For this review, take the finished solid that the model builds, in its own axes (mm). A direction names the side the tool comes from. Give positions to 0.01 mm unless a question says otherwise; leave off trailing zeros. Loops run counter-clockwise (first coordinate to the right, second up) from the corner with the lowest first, then second, coordinate; pieces in that order, holes last. Notation, with made-up numbers: (-36.75, 33.25) - (6.25, 33.25) arc R16 cw to (6.25, 53.25) - close; hole circle Ø11 at (81.5, 23). An arc over 180 degrees is marked (long way). Answer in a Markdown table with one row per item.
```python
from build123d import *

# Parameters (mm, degrees)
F0_W     = 20
F0_H     = 20
F1_DEPTH = 10
F2_R     = 2.5
F3_DEPTH = 2
F4_R     = 2.5
F5_DEPTH = 2
F6_R     = 2.5
F7_DEPTH = 2
F8_R     = 1.5


# Not quite as in the source:
# - a pattern or mirror of a feature is missing from the dataset's text; its kind, count and spacing are read off the source's solid


with BuildPart() as f1:
    # F0 (on Top) → F1 (new body, symmetric)
    with BuildSketch(Plane.XY):
        Rectangle(F0_W, F0_H)
    extrude(amount=F1_DEPTH, both=True)

    # F2 (on face) → F3 (cut)
    with BuildSketch(Plane.YZ.offset(10)):
        Circle(F2_R)
    f3 = extrude(amount=-F3_DEPTH, mode=Mode.SUBTRACT)

    # F3_copies: F3 across plane
    add(f3.mirror(Plane(origin=(0, 0, 0), x_dir=(0, 0, -1), z_dir=(-1, 0, 0))), mode=Mode.SUBTRACT)

    # F4 (on face) → F5 (cut)
    with BuildSketch(Plane(origin=(0, 10, 0), x_dir=(-1, 0, 0), z_dir=(0, 1, 0))):
        with Locations((5, -5)):
            Circle(F4_R)
        with Locations((-5, 5)):
            Circle(F4_R)
    extrude(amount=-F5_DEPTH, mode=Mode.SUBTRACT)

    # F6 (on face) → F7 (cut)
    with BuildSketch(Plane.XZ.offset(10)):
        with Locations((-5, 5)):
            Circle(F6_R)
        with Locations((5, -5)):
            Circle(F6_R)
    extrude(amount=-F7_DEPTH, mode=Mode.SUBTRACT)

    # F8
    f8_edges = [f1.edges().sort_by_distance(p)[0] for p in [
        (10, 0, 10),
        (0, 10, 10),
        (10, 10, 0),
        (10, -10, 0),
        (10, 0, -10),
        (0, -10, -10),
        (-10, 0, -10),
        (0, 10, -10),
        (-10, 10, 0),
        (-10, -10, 0),
        (0, -10, 10),
        (-10, 0, 10),
    ]]
    fillet(f8_edges, radius=F8_R)


solid = f1.part
```
1. Mouldability with a two-part tool opening along X and no side actions: class faces 6 (the face through (5, 8, 5)), 7 (the face through (9.55, 0.12, 9.57)), 8 (the face through (-10, -2, 2)), 9 (the face through (-2.615, -9.014, 5.751)) as released by +X, released by -X, zero draft, split by the parting line, or undercut.
Values:
| item | result |
|---|---|
| face 6 | undercut |
| face 7 | released by +X |
| face 8 | released by -X |
| face 9 | undercut |
2. Clearance check with flat-ended pins moving along their axes: pin 1 (1.5 mm diameter, centred on x = 6, z = -5.5, fed in from -Y); pin 2 (8 mm diameter, centred on x = 4, z = -6, fed in from -Y); pin 3 (2.5 mm diameter, centred on x = -5, z = -5, fed in from +Y); pin 4 (2.5 mm diameter, centred on y = 0, z = -1, fed in from +X). State where each tip first meets the part, or that it passes through.
Values:
| item | result |
|---|---|
| pin 1 | stops at y = -8 |
| pin 2 | stops at y = -10 |
| pin 3 | stops at y = 8 |
| pin 4 | stops at x = 8 |
3. Wall thickness on line 1 (Y direction, x = -5, z = -5.5); line 2 (Z direction, x = 9.3, y = 0); line 3 (Z direction, x = -9, y = 0.75): over which ranges is each line inside the solid? List them lowest first. Write a range as [from, to].
Values:
| item | result |
|---|---|
| line 1 | y = [-10, 8] |
| line 2 | z = [-9.77, -2.5], [2.5, 9.77] |
| line 3 | z = [-9.91, -2.38], [2.38, 9.91] |
4. For faces 1 (the face through (-7.385, 9.014, -4.249)), 2 (the face through (-5, -8, 5)), 3 (the face through (0, -10, 0)), 4 (the face through (9.55, -9.57, 0.12)), 5 (the face through (8, 0, 0)), list the 3-axis set-ups (+Z, -Z, +X, -X, +Y, -Y) from which the entire face can be reached by the end or side of a thin tool; tool diameter is ignored.
Values:
| item | result |
|---|---|
| face 1 | +Y |
| face 2 | -Y |
| face 3 | +Z, -Z, +X, -X, -Y |
| face 4 | +Z, -Z, +X, -Y |
| face 5 | +X |
5. We need section A-A, the plane z = 3.5. Give the boundary of the cut face in (x, y).
Values:
| item | result |
|---|---|
| outline | (-10, -8.5) arc R1.5 ccw to (-8.5, -10) - (-7, -10) - (-7, -8) - (-3, -8) - (-3, -10) - (8.5, -10) arc R1.5 ccw to (10, -8.5) - (10, 8.5) arc R1.5 ccw to (8.5, 10) - (7, 10) - (7, 8) - (3, 8) - (3, 10) - (-8.5, 10) arc R1.5 ccw to (-10, 8.5) - close |
6. We need section B-B, the plane y = 0. Give the boundary of the cut face in (x, z).
Values:
| item | result |
|---|---|
| outline | (-10, -8.5) arc R1.5 ccw to (-8.5, -10) - (8.5, -10) arc R1.5 ccw to (10, -8.5) - (10, -2.5) - (8, -2.5) - (8, 2.5) - (10, 2.5) - (10, 8.5) arc R1.5 ccw to (8.5, 10) - (-8.5, 10) arc R1.5 ccw to (-10, 8.5) - (-10, 2.5) - (-8, 2.5) - (-8, -2.5) - (-10, -2.5) - close |
